Answer from the drawing. Dimensions are ordinates in mm from the lowest x, y and z of the part. Coordinates: 2 decimals unless noted, no trailing zeros. Loops run counter-clockwise (first coordinate to the right, second up) from the corner with the lowest first, then second, coordinate; pieces in that order, holes last. Notation, with made-up numbers: M 53.5,57 L 66.5,57 A35 ccw 66.5,90 Z; hole C -40,50 d1. An arc over 180 degrees is marked long. Answer as CSV lines item,"result". Start each with the question number.
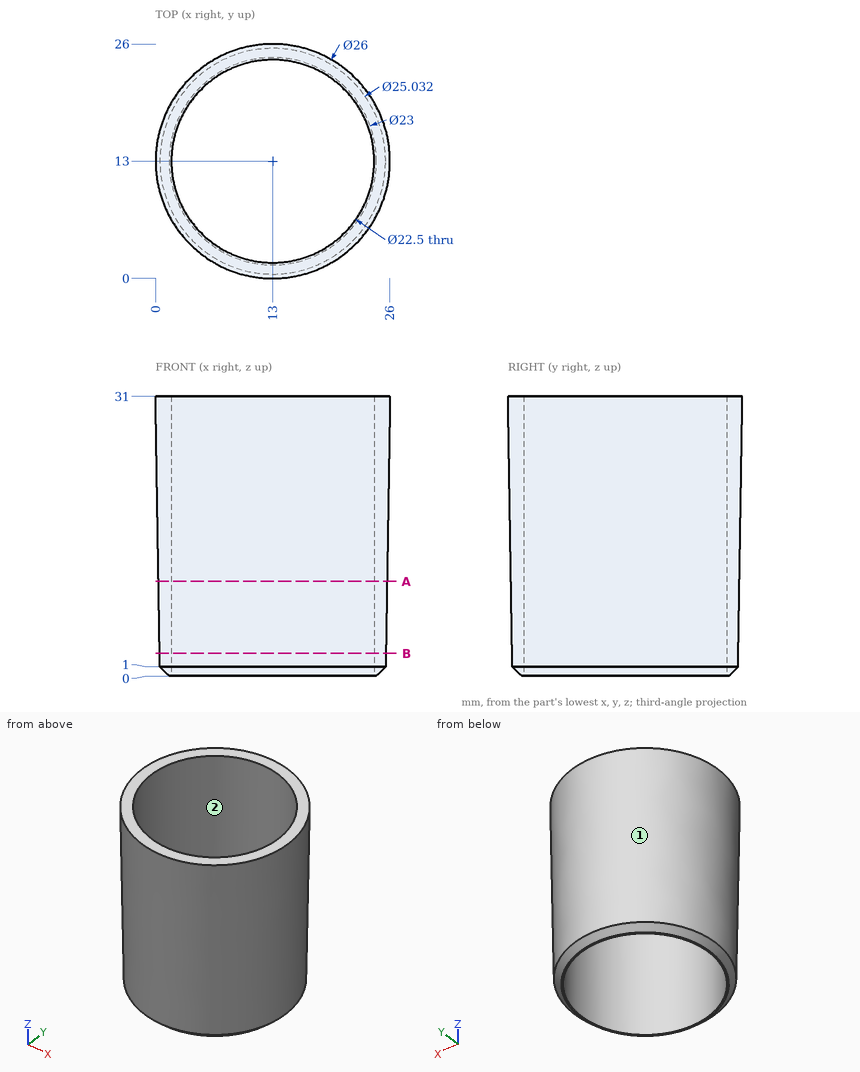
Item 1: Consider line 1 (Y direction, x = 5, z = 22); line 2 (Y direction, x = 11.5, z = 26.5); line 3 (X direction, y = 20.25, z = 21.5) (1 decimal). Determine where each line is inside the solid, lowest interval first.
Item 2: Section A-A on z = 10.5 is taken. Determine the outline of the cut face in (x, y).
Item 3: Each of these flat-tipped pins is pushed along its axis until it touches: P1, Ø2, axis at y = 18.5, z = 7, coming from the -X side; P2, Ø5, axis at x = 2.5, z = 16.5, coming from the -Y side; P3, Ø1, axis at y = 20.5, z = 6, coming from the -X side; P4, Ø12, axis at x = 18, y = 22.5, coming from the +Z side. Where does it stop, or does it pass through?
Item 4: Section B-B on z = 2.5 is taken. Determine the outline of the cut face in (x, y).
Item 5: For a pull along X with two mould halves and no side action, classify the marked faces 1 and 2 as pulls with the +X half, pulls with the -X half, needs draft (parallel to the pull), parting line crosses it, or undercut.
Results are:
1,line 1,"2.94 to 5.09, 20.91 to 23.06"
1,line 2,"0.16 to 1.85, 24.15 to 25.84"
1,line 3,"2.4 to 4.4, 21.6 to 23.6"
2,outline,"C 13,13 d25.34; hole C 13,13 d22.5"
3,P1,"x = 1.22"
3,P2,"y = 3.05"
3,P3,"x = 2.53"
3,P4,"z = 31"
4,outline,"C 13,13 d25.08; hole C 13,13 d22.5"
5,face 1,"parting line crosses it"
5,face 2,"undercut"
